Part model, mm, in its own coordinate system. A direction names the side the tool comes from. Coordinates: 2 decimals unless noted, no trailing zeros. One line per question, with ' | ' between items. Start each with the question number.
1) Drop flat-ended pins along their axis: pin 1 (0.6 mm diameter, centred on x = 11.5, z = -2, fed in from +Y); pin 2 (1.1 mm diameter, centred on x = 24, y = 4, fed in from +Z); pin 3 (0.6 mm diameter, centred on y = 0, z = -1.5, fed in from -X); pin 4 (0.5 mm diameter, centred on x = 8, y = 2, fed in from +Z). Give the stop position or say it passes through.
2) Two-plate mould, pull along Y, no slides. Class faces 1 (the face through (11.6, 2.3, 7.5)), 2 (the face through (0, 3, 5)), 3 (the face through (13, 0, 3)), 4 (the face through (22.477, 2.15, 7.535)): released by +Y, released by -Y, zero draft, split by the parting line, or undercut.
3) Cut at A-A (z = 7.25). Count the separate pieces of the cut face and the enclosed holes in it, plus the area to 3 significant figures.
4) 3-axis set-ups, long thin cutter, end or side, ignore diameter. For faces 5 (the face through (6, 2, 5)), 6 (the face through (13, 3, 10)): which of +Z, -Z, +X, -X, +Y, -Y reach the whole face in a straight line?
5) Probe L1, parallel to Y at x = 12, z = 8.5; L2, parallel to Z at x = 4.25, y = 5.65; L3, parallel to Z at x = 6.25, y = 1.65. List the from-to ranges inside material, lowest first. Write a range as from..to.
from build123d import *

# Parameters (mm, degrees)
SKETCH2_W           = 26
SKETCH2_H           = 6
BOSS_EXTRUDE1_DEPTH = 10
SKETCH3_R           = 0.5
CUT_EXTRUDE1_DEPTH  = 5
SKETCH4_W           = 0.5
SKETCH4_H           = 3
BOSS_EXTRUDE2_DEPTH = 0.5


with BuildPart() as part:
    # Sketch2 → Boss-Extrude1 (new body)
    with BuildSketch(Plane.XY):
        with Locations((13, 3)):
            Rectangle(SKETCH2_W, SKETCH2_H)
    extrude(amount=BOSS_EXTRUDE1_DEPTH)

    # Sketch3 → Cut-Extrude1 (cut)
    with BuildSketch(Plane.XY.offset(10)):
        with Locations((2, 2)):
            Circle(SKETCH3_R)
        with Locations((4, 2)):
            Circle(SKETCH3_R)
        with Locations((6, 2)):
            Circle(SKETCH3_R)
        with Locations((8, 2)):
            Circle(SKETCH3_R)
        with Locations((10, 2)):
            Circle(SKETCH3_R)
        with Locations((12, 2)):
            Circle(SKETCH3_R)
        with Locations((14, 2)):
            Circle(SKETCH3_R)
        with Locations((16, 2)):
            Circle(SKETCH3_R)
        with Locations((18, 2)):
            Circle(SKETCH3_R)
        with Locations((20, 2)):
            Circle(SKETCH3_R)
        with Locations((22, 2)):
            Circle(SKETCH3_R)
        with Locations((24, 2)):
            Circle(SKETCH3_R)
        with Locations((24, 4)):
            Circle(SKETCH3_R)
        with Locations((22, 4)):
            Circle(SKETCH3_R)
        with Locations((20, 4)):
            Circle(SKETCH3_R)
        with Locations((18, 4)):
            Circle(SKETCH3_R)
        with Locations((16, 4)):
            Circle(SKETCH3_R)
        with Locations((14, 4)):
            Circle(SKETCH3_R)
        with Locations((12, 4)):
            Circle(SKETCH3_R)
        with Locations((10, 4)):
            Circle(SKETCH3_R)
        with Locations((8, 4)):
            Circle(SKETCH3_R)
        with Locations((6, 4)):
            Circle(SKETCH3_R)
        with Locations((4, 4)):
            Circle(SKETCH3_R)
        with Locations((2, 4)):
            Circle(SKETCH3_R)
    extrude(amount=-CUT_EXTRUDE1_DEPTH, mode=Mode.SUBTRACT)

    # Sketch4 → Boss-Extrude2 (add)
    with BuildSketch(Plane(origin=(0, 0, 0), x_dir=(-1, 0, 0), z_dir=(0, -1, 0))):
        with Locations((-24.65, 1.5)):
            Rectangle(SKETCH4_W, SKETCH4_H)
        with Locations((-25.75, 1.5)):
            Rectangle(SKETCH4_W, SKETCH4_H)
        with Locations((-23.55, 1.5)):
            Rectangle(SKETCH4_W, SKETCH4_H)
        with Locations((-22.45, 1.5)):
            Rectangle(SKETCH4_W, SKETCH4_H)
        with Locations((-21.35, 1.5)):
            Rectangle(SKETCH4_W, SKETCH4_H)
        with Locations((-20.25, 1.5)):
            Rectangle(SKETCH4_W, SKETCH4_H)
        with Locations((-19.15, 1.5)):
            Rectangle(SKETCH4_W, SKETCH4_H)
        with Locations((-18.05, 1.5)):
            Rectangle(SKETCH4_W, SKETCH4_H)
        with Locations((-16.95, 1.5)):
            Rectangle(SKETCH4_W, SKETCH4_H)
        with Locations((-15.85, 1.5)):
            Rectangle(SKETCH4_W, SKETCH4_H)
        with Locations((-14.75, 1.5)):
            Rectangle(SKETCH4_W, SKETCH4_H)
        with Locations((-13.65, 1.5)):
            Rectangle(SKETCH4_W, SKETCH4_H)
        with Locations((-12.55, 1.5)):
            Rectangle(SKETCH4_W, SKETCH4_H)
        with Locations((-11.45, 1.5)):
            Rectangle(SKETCH4_W, SKETCH4_H)
        with Locations((-10.35, 1.5)):
            Rectangle(SKETCH4_W, SKETCH4_H)
        with Locations((-9.25, 1.5)):
            Rectangle(SKETCH4_W, SKETCH4_H)
        with Locations((-8.15, 1.5)):
            Rectangle(SKETCH4_W, SKETCH4_H)
        with Locations((-7.05, 1.5)):
            Rectangle(SKETCH4_W, SKETCH4_H)
        with Locations((-5.95, 1.5)):
            Rectangle(SKETCH4_W, SKETCH4_H)
        with Locations((-4.85, 1.5)):
            Rectangle(SKETCH4_W, SKETCH4_H)
        with Locations((-3.75, 1.5)):
            Rectangle(SKETCH4_W, SKETCH4_H)
        with Locations((-2.65, 1.5)):
            Rectangle(SKETCH4_W, SKETCH4_H)
        with Locations((-1.55, 1.5)):
            Rectangle(SKETCH4_W, SKETCH4_H)
        with Locations((-0.45, 1.5)):
            Rectangle(SKETCH4_W, SKETCH4_H)
    extrude(amount=-BOSS_EXTRUDE2_DEPTH)


solid = part.part
Reported:
1) pin 1: stops at y = 0.5 | pin 2: stops at z = 10 | pin 3: stops at x = 0.2 | pin 4: stops at z = 5
2) face 1: undercut | face 2: zero draft | face 3: released by -Y | face 4: undercut
3) separate pieces: 1 | enclosed holes: 24 | area: 137 mm²
4) face 5: +Z | face 6: +Z, +X, -X, +Y, -Y
5) L1: y = 0..1.5, 2.5..3.5, 4.5..6 | L2: z = 0..10 | L3: z = 0..5
